from build123d import *

# Parameters (mm, degrees)
EXTRUDE_1_DEPTH          = 3
CUT_EXTRUDE_2_REACH      = 99.793
SKETCH_3_R               = 1.6
PATTERN_LINEAR_1_COUNT   = 4
PATTERN_LINEAR_1_PITCH   = 15
CUT_EXTRUDE_1_REACH      = 99.793
SKETCH_2_R               = 1.5
PATTERN_CIRCULAR_1_COUNT = 4


with BuildPart() as part:
    # Sketch 1 → Extrude 1 (new body)
    with BuildSketch(Plane.XY):
        with BuildLine():
            Line((-28.5, 0), (28.5, 0))
            Line((28.5, 0), (28.5, -65))
            ThreePointArc((28.5, -65), (0, -93.5), (-28.5, -65))
            Line((-28.5, -65), (-28.5, 0))
        make_face()
    extrude(amount=EXTRUDE_1_DEPTH)

    # Sketch 3 → Cut-Extrude 2 (cut, up to next)
    with BuildSketch(Plane.XY.offset(3), mode=Mode.PRIVATE) as cut_extrude_2_sk1:
        with Locations((-22.5, -4)):
            Circle(SKETCH_3_R)
    cut_extrude_2_tool1 = extrude(cut_extrude_2_sk1.sketch, amount=-CUT_EXTRUDE_2_REACH, mode=Mode.PRIVATE) & part.part
    cut_extrude_2 = cut_extrude_2_tool1.solids().sort_by_distance((-22.5, -4, 3))[0]
    add(cut_extrude_2, mode=Mode.SUBTRACT)

    # Pattern Linear 1: Cut-Extrude 2 ×4
    with Locations(*[(i * PATTERN_LINEAR_1_PITCH, 0, 0) for i in range(1, PATTERN_LINEAR_1_COUNT)]):
        add(cut_extrude_2, mode=Mode.SUBTRACT)

    # Sketch 2 → Cut-Extrude 1 (cut, up to next)
    with BuildSketch(Plane.XY.offset(3), mode=Mode.PRIVATE) as cut_extrude_1_sk1:
        with Locations((-6, -53)):
            Circle(SKETCH_2_R)
    cut_extrude_1_tool1 = extrude(cut_extrude_1_sk1.sketch, amount=-CUT_EXTRUDE_1_REACH, mode=Mode.PRIVATE) & part.part
    # Sketch 2 → Cut-Extrude 1 (cut, up to next)
    with BuildSketch(Plane.XY.offset(3), mode=Mode.PRIVATE) as cut_extrude_1_sk2:
        with Locations((-12, -59)):
            Circle(SKETCH_2_R)
    cut_extrude_1_tool2 = extrude(cut_extrude_1_sk2.sketch, amount=-CUT_EXTRUDE_1_REACH, mode=Mode.PRIVATE) & part.part
    cut_extrude_1_1 = cut_extrude_1_tool1.solids().sort_by_distance((-6, -53, 3))[0]
    add(cut_extrude_1_1, mode=Mode.SUBTRACT)
    cut_extrude_1_2 = cut_extrude_1_tool2.solids().sort_by_distance((-12, -59, 3))[0]
    add(cut_extrude_1_2, mode=Mode.SUBTRACT)
    cut_extrude_1 = cut_extrude_1_1 + cut_extrude_1_2  # Cut-Extrude 1 as one shape, for the pattern or mirror that repeats it

    # Pattern Circular 1: Cut-Extrude 1 ×4 about axis
    pattern_circular_1_axis = Axis((0, -65, 0), (0, 0, 1))
    for i in range(1, PATTERN_CIRCULAR_1_COUNT):
        add(cut_extrude_1.rotate(pattern_circular_1_axis, i * 360 / PATTERN_CIRCULAR_1_COUNT), mode=Mode.SUBTRACT)


solid = part.part
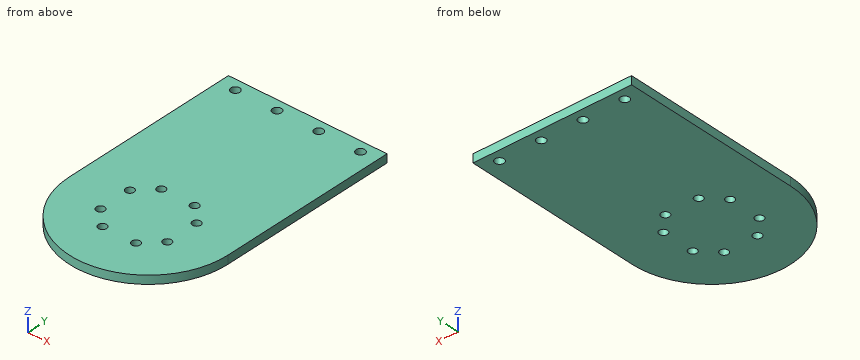
Source: CAD feature listing. Evaluate the final solid. Frame: model axes, mm. Round coordinates to 2 decimals unless told otherwise and drop trailing zeros. Loops run counter-clockwise (first coordinate to the right, second up) from the corner with the lowest first, then second, coordinate; pieces in that order, holes last. Notation, with made-up numbers: (-14.5, -32) - (26.5, -32) arc R31 ccw to (26.5, -2) - close; hole circle Ø4 at (42, -36.75). An arc over 180 degrees is marked (long way). Write item = value, one per line. Start each with the question number.
Item 1: Section query C-C on x = -12. Output: boundary loops of the cut face in (y, z).
Item 2: First-contact query: pin 1 Ø1 at (x, z) = (5, 1.5) entering from -Y. Flat tip, straight axial feed; report the tip coordinate or a pass-through.
Item 3: Section query B-B on x = -22.5. Output: boundary loops of the cut face in (y, z), plus the area to 3 significant figures.
Item 4: Material intervals for line 1 (X direction, y = -53, z = 1.7); line 2 (X direction, y = -59, z = 1.6); line 3 (Y direction, x = -12, z = 1.8), sorted ascending.
Item 5: Section query A-A on z = 1.6. Count the separate pieces of the cut face and the enclosed holes in it, plus the area to 3 significant figures.
Item 6: Section query D-D on y = -85. Output: boundary loops of the cut face in (x, z), plus the area to 3 significant figures.
Results list:
q1.outline = (-90.85, 0) - (-72.5, 0) - (-72.5, 3) - (-90.85, 3) - close; (-69.5, 0) - (-60.5, 0) - (-60.5, 3) - (-69.5, 3) - close; (-57.5, 0) - (0, 0) - (0, 3) - (-57.5, 3) - close
q2.pin_1 = -93.14
q3.outline = (-82.49, 0) - (-5.6, 0) - (-5.6, 3) - (-82.49, 3) - close; (-2.4, 0) - (0, 0) - (0, 3) - (-2.4, 3) - close
q3.area = 238 mm²
q4.line_1 = -28.5 to -7.5, -4.5 to 4.5, 7.5 to 28.5
q4.line_2 = -28.5 to -13.5, -10.5 to 10.5, 13.5 to 28.5
q4.line_3 = -90.85 to -72.5, -69.5 to -60.5, -57.5 to 0
q5.separate_pieces = 1
q5.enclosed_holes = 12
q5.area = 4,890 mm²
q6.outline = (-20.3, 0) - (20.3, 0) - (20.3, 3) - (-20.3, 3) - close
q6.area = 122 mm²
